Verification items for the finished model (mm, model axes). Face numbers are marked on the shaded views. A direction names the side the tool comes from. Coordinates: 2 decimals unless noted, no trailing zeros. Order: outer loops, then holes, each group sorted by start corner. A loop starts at its lowest first (then second) coordinate and runs counter-clockwise, first axis right, second up. Notation, with made-up numbers: (6.5, -1) -> (25.5, -1) arc R19 ccw to (25.5, 5) -> close; hole circle Ø7 at (-28.75, 16.5). An arc over 180 degrees is marked (long way). Write each question's results on one line, items separated by ' | '. Start each with the question number.
(1) Set-up check for the marked faces 5 and 6: record each of +Z, -Z, +X, -X, +Y, -Y from which the full face is reachable in a straight line by a thin tool's end or side.
(2) Thickness scan on probe 1 along X at (y, z) = (49.2, 49.5); probe 2 along Y at (x, z) = (0.5, 40.5); probe 3 along Z at (x, y) = (0, 48.75). Record the ranges inside material, lowest first. Write a range as [from, to].
(3) Cross-section at B-B on z = 49.5. Enter the section's corners in (x, y), and give its area (3 significant figures).
(4) Cross-section at D-D on z = 40.5. Enter the section's corners in (x, y), and give its area (3 significant figures).
(5) Go/stop test with flat-tipped pins: pin 1 (4 mm diameter, centred on x = 12, z = 51, fed in from -Y); pin 2 (4 mm diameter, centred on x = 7.5, y = 50.5, fed in from -Z); pin 3 (6 mm diameter, centred on x = -5.5, y = 41, fed in from -Z). Record where each tip stops, or that it passes through.
(6) Cross-section at C-C on y = 49.75. Enter the section's corners in (x, z), and give its area (3 significant figures).
(7) Draft check along X on the marked faces 1, 2, 3 and 4. Enter one of: +X half, -X half, draft (parallel to the pull), parting line (faces both ways), or undercut.
(8) Cross-section at A-A on x = 0. Enter the section's corners in (y, z).
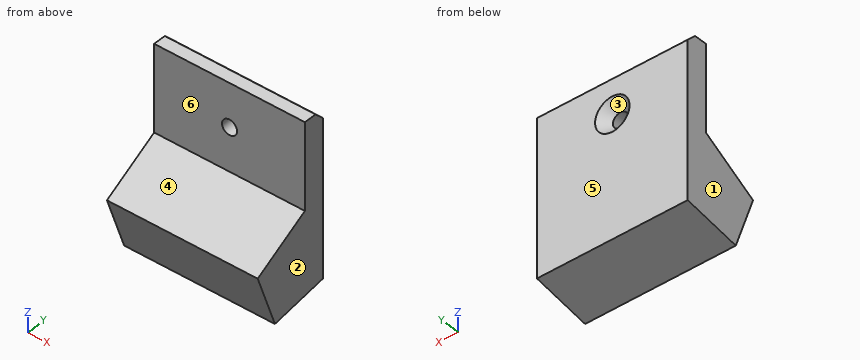
```python
from build123d import *

# Parameters (mm, degrees)
PAD_DEPTH        = 17.5
HOLE_D           = 3.5
HOLE_CSINK_D     = 8
HOLE_CSINK_ANGLE = 90


with BuildPart() as part:
    # Sketch → Pad (new body, symmetric)
    with BuildSketch(Plane.YZ):
        Polygon((34.641016, 32), (47.631397, 39.5), (47.631397, 59.5), (50.560329, 59.5), (52.631397, 57.428932), (52.631397, 21.280335), (39.39231, 18.945927), align=None)
    extrude(amount=PAD_DEPTH, both=True)

    # Hole (through all)
    with Locations(Plane.ZX.offset(52.631397)):
        with Locations((49.5, 0)):
            CounterSinkHole(HOLE_D / 2, HOLE_CSINK_D / 2, counter_sink_angle=HOLE_CSINK_ANGLE)


solid = part.part
```
Results are:
1) face 5: +Z, -Z, +X, -X, +Y | face 6: +Z, +X, -X, -Y
2) probe 1: x = [-17.5, -1.75], [1.75, 17.5] | probe 2: y = [47.63, 52.63] | probe 3: z = [20.6, 47.75], [51.25, 59.5]
3) outline: (-17.5, 47.63) -> (-1.75, 47.63) -> (-1.75, 50.38) -> (-4, 52.63) -> (-17.5, 52.63) -> close; (1.75, 47.63) -> (17.5, 47.63) -> (17.5, 52.63) -> (4, 52.63) -> (1.75, 50.38) -> close | area: 152 mm2
4) outline: (-17.5, 47.63) -> (17.5, 47.63) -> (17.5, 52.63) -> (-17.5, 52.63) -> close | area: 175 mm2
5) pin 1: stops at y = 47.63 | pin 2: stops at z = 20.55 | pin 3: stops at z = 18.95
6) outline: (-17.5, 20.77) -> (17.5, 20.77) -> (17.5, 59.5) -> (-17.5, 59.5) -> close; hole circle Ø3.5 at (0, 49.5) | area: 1,350 mm2
7) face 1: -X half | face 2: +X half | face 3: undercut | face 4: draft
8) outline: (34.64, 32) -> (39.39, 18.95) -> (52.63, 21.28) -> (52.63, 45.5) -> (50.38, 47.75) -> (47.63, 47.75) -> (47.63, 39.5) -> close; (47.63, 51.25) -> (50.38, 51.25) -> (52.63, 53.5) -> (52.63, 57.43) -> (50.56, 59.5) -> (47.63, 59.5) -> close
